CAD build for the part. Positions are in the model's coordinates, mm. Face numbers are marked on the shaded views. Give positions to 0.01 mm unless a question says otherwise; leave off trailing zeros. Loops run counter-clockwise (first coordinate to the right, second up) from the corner with the lowest first, then second, coordinate; pieces in that order, holes last. Notation, with made-up numbers: M 25.5,-29 L 33.5,-29 A23 ccw 33.5,-11 Z; hole C 7.25,78 d6. An arc over 180 degrees is marked long. Answer as CSV lines item,"result".
```python
from build123d import *

# Parameters (mm, degrees)
SKETCH1_W           = 154
SKETCH1_H           = 67
SKETCH1_R           = 4
SKETCH1_W_2         = 98.2
SKETCH1_H_2         = 40.7
BOSS_EXTRUDE1_DEPTH = 2
SKETCH2_R           = 4
SKETCH2_R_2         = 1.3
BOSS_EXTRUDE2_DEPTH = 10.2
BOSS_EXTRUDE3_DEPTH = 3
BOSS_EXTRUDE4_DEPTH = 3
SKETCH4_R           = 1.7
CUT_EXTRUDE1_DEPTH  = 2


with BuildPart() as part:
    # Sketch1 → Boss-Extrude1 (new body)
    with BuildSketch(Plane(origin=(0, 0, -3.9), x_dir=(-1, 0, 0), z_dir=(0, 0, -1))):
        Rectangle(SKETCH1_W, SKETCH1_H)
        with Locations((-61.7, -15.35)):
            Circle(SKETCH1_R, mode=Mode.SUBTRACT)
        with Locations((-62.3, 2.75)):
            Circle(SKETCH1_R, mode=Mode.SUBTRACT)
        with BuildLine():
            Line((-57.130294851, 15.75), (-65.269705149, 15.75))
            ThreePointArc((-65.269705149, 15.75), (-66.019705149, 15), (-65.269705149, 14.25))
            Line((-65.269705149, 14.25), (-57.130294851, 14.25))
            ThreePointArc((-57.130294851, 14.25), (-56.380294851, 15), (-57.130294851, 15.75))
        make_face(mode=Mode.SUBTRACT)
        with BuildLine():
            Line((-65.269705149, 27.75), (-57.130294851, 27.75))
            ThreePointArc((-57.130294851, 27.75), (-56.380294851, 27), (-57.130294851, 26.25))
            Line((-57.130294851, 26.25), (-65.269705149, 26.25))
            ThreePointArc((-65.269705149, 26.25), (-66.019705149, 27), (-65.269705149, 27.75))
        make_face(mode=Mode.SUBTRACT)
        with BuildLine():
            Line((-68.45, 21.75), (-53.95, 21.75))
            ThreePointArc((-53.95, 21.75), (-53.2, 21), (-53.95, 20.25))
            Line((-53.95, 20.25), (-68.45, 20.25))
            ThreePointArc((-68.45, 20.25), (-69.2, 21), (-68.45, 21.75))
        make_face(mode=Mode.SUBTRACT)
        with BuildLine():
            Line((-54.599810609, 18.75), (-67.800189391, 18.75))
            ThreePointArc((-67.800189391, 18.75), (-68.550189391, 18), (-67.800189391, 17.25))
            Line((-67.800189391, 17.25), (-54.599810609, 17.25))
            ThreePointArc((-54.599810609, 17.25), (-53.849810609, 18), (-54.599810609, 18.75))
        make_face(mode=Mode.SUBTRACT)
        with BuildLine():
            Line((-54.599810609, 23.25), (-67.800189391, 23.25))
            ThreePointArc((-67.800189391, 23.25), (-68.550189391, 24), (-67.800189391, 24.75))
            Line((-67.800189391, 24.75), (-54.599810609, 24.75))
            ThreePointArc((-54.599810609, 24.75), (-53.849810609, 24), (-54.599810609, 23.25))
        make_face(mode=Mode.SUBTRACT)
        with Locations((12.7, -1.35)):
            Rectangle(SKETCH1_W_2, SKETCH1_H_2, mode=Mode.SUBTRACT)
    extrude(amount=-BOSS_EXTRUDE1_DEPTH)

    # Sketch2 → Boss-Extrude2 (add)
    with BuildSketch(Plane(origin=(0, 0, -3.9), x_dir=(-1, 0, 0), z_dir=(0, 0, -1))):
        with Locations((-72.25, 28.75)):
            Circle(SKETCH2_R)
        with Locations((-72.25, 28.75)):
            Circle(SKETCH2_R_2, mode=Mode.SUBTRACT)
        with Locations((-72.25, -20.75)):
            Circle(SKETCH2_R)
        with Locations((-72.25, -20.75)):
            Circle(SKETCH2_R_2, mode=Mode.SUBTRACT)
        with Locations((72.25, -20.75)):
            Circle(SKETCH2_R)
        with Locations((72.25, -20.75)):
            Circle(SKETCH2_R_2, mode=Mode.SUBTRACT)
        with Locations((72.25, 28.75)):
            Circle(SKETCH2_R)
        with Locations((72.25, 28.75)):
            Circle(SKETCH2_R_2, mode=Mode.SUBTRACT)
    extrude(amount=BOSS_EXTRUDE2_DEPTH)

    # Sketch3 → Boss-Extrude3 (add, symmetric)
    with BuildSketch(Plane.ZY.offset(72.25)):
        Polygon((-7.4, 35.55), (-3.9, 30.05), (-14.1, 30.05), (-14.1, 35.55), align=None)
    extrude(amount=BOSS_EXTRUDE3_DEPTH, both=True)

    # Sketch5 → Boss-Extrude4 (add, symmetric)
    with BuildSketch(Plane(origin=(72.25, 0, 0), x_dir=(0, 0, -1), z_dir=(1, 0, 0))):
        Polygon((3.9, 30.05), (7.4, 35.55), (14.1, 35.55), (14.1, 30.05), align=None)
    extrude(amount=BOSS_EXTRUDE4_DEPTH, both=True)

    # Sketch4 → Cut-Extrude1 (cut)
    with BuildSketch(Plane.XY.offset(-1.9)):
        with Locations((-70.376631043, -28.876631043)):
            Circle(SKETCH4_R)
        with Locations((70.376631043, -28.876631043)):
            Circle(SKETCH4_R)
    extrude(amount=-CUT_EXTRUDE1_DEPTH, mode=Mode.SUBTRACT)


solid = part.part
```
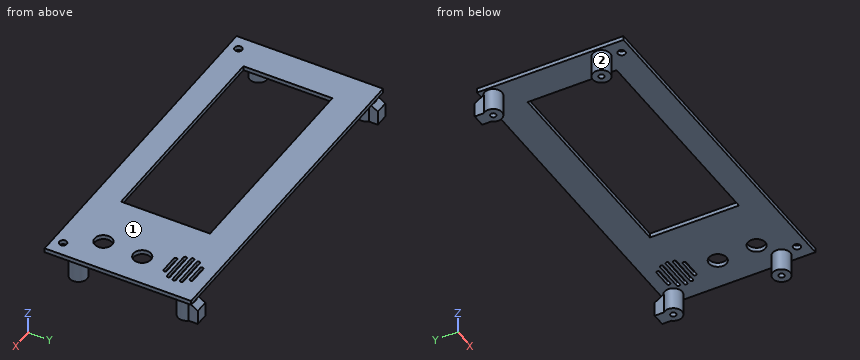
Q1. Cut at C-C (y = 2.75). Write the cut outline in (x, z).
Solution:
outline,"M -77,-3.9 L -61.8,-3.9 L -61.8,-1.9 L -77,-1.9 Z; M 36.4,-3.9 L 58.3,-3.9 L 58.3,-1.9 L 36.4,-1.9 Z; M 66.3,-3.9 L 77,-3.9 L 77,-1.9 L 66.3,-1.9 Z"
Q2. Pin check, flat tips, straight feed: P1, Ø4, axis at x = -70.38, y = -28.88, coming from the -Z side; P2, Ø0.6, axis at x = 7, z = -3.5, coming from the +Y side; P3, Ø6, axis at y = -24, z = -11, coming from the -X side. Stop position of each tip, or through.
Solution:
P1,"stops at z = -3.9"
P2,"stops at y = 33.5"
P3,"stops at x = -76.24"
Q3. Cut at D-D (x = -24.5). Write the cut outline in (y, z), and give its area (3 significant figures).
Solution:
outline,"M -33.5,-3.9 L -21.7,-3.9 L -21.7,-1.9 L -33.5,-1.9 Z; M 19,-3.9 L 33.5,-3.9 L 33.5,-1.9 L 19,-1.9 Z"
area,"52.6 mm²"
Q4. Wall check: line 1 (Y direction, x = 72.25, z = -8); line 2 (X direction, y = -29, z = -3.25); line 3 (X direction, y = -20.5, z = -3). Give the ranges that are in metal, low to high. Write a range as [from, to].
Solution:
line 1,"y = [-24.75, -22.05], [-19.45, -16.75], [24.75, 27.45], [30.05, 35.55]"
line 2,"x = [-77, -72.07], [-68.68, 68.68], [72.07, 77]"
line 3,"x = [-77, -61.8], [36.4, 77]"
Q5. Cut at A-A (z = -9.5). Write the cut outline in (x, y).
Solution:
outline,"C -72.25,-20.75 d8; M -75.25,31.4 A4 ccw long -69.25,31.4 L -69.25,35.55 L -75.25,35.55 Z; C 72.25,-20.75 d8; M 69.25,31.4 A4 ccw long 75.25,31.4 L 75.25,35.55 L 69.25,35.55 Z; hole C -72.25,-20.75 d2.6; hole C -72.25,28.75 d2.6; hole C 72.25,-20.75 d2.6; hole C 72.25,28.75 d2.6"
Q6. Cut at B-B (y = -4.5). Write the cut outline in (x, z), and give its area (3 significant figures).
Solution:
outline,"M -77,-3.9 L -61.8,-3.9 L -61.8,-1.9 L -77,-1.9 Z; M 36.4,-3.9 L 77,-3.9 L 77,-1.9 L 36.4,-1.9 Z"
area,"112 mm²"
Q7. Mould opens along X. For the marked faces 1 and 2 say: released by +X, released by -X, zero draft, split by the parting line, or undercut.
Solution:
face 1,"zero draft"
face 2,"undercut"
